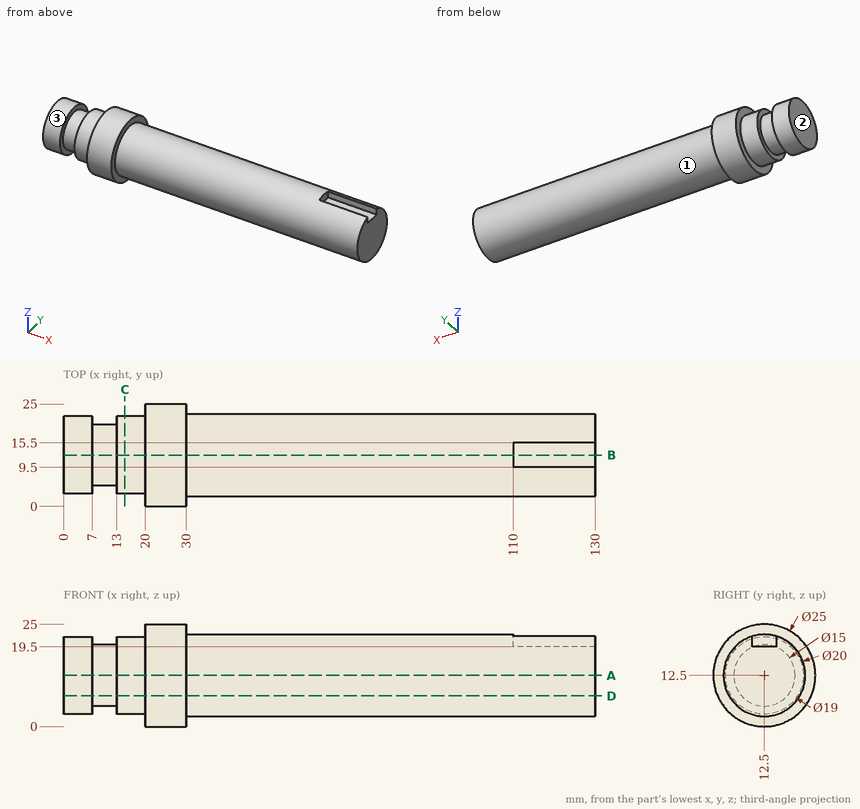
Here's the drawing with two shaded views (mm, measured from the low corner). I have some questions. A direction names the side the tool comes from. Coordinates: 2 decimals unless noted, no trailing zeros. Order: outer loops, then holes, each group sorted by start corner. A loop starts at its lowest first (then second) coordinate and runs counter-clockwise, first axis right, second up. Notation, with made-up numbers: (73.5, -23.5) - (84.5, -23.5) arc R28 ccw to (84.5, -1.5) - close; hole circle Ø4 at (86, 81.25). An arc over 180 degrees is marked (long way). Answer in a Markdown table with one row per item. Add a question column.
(1) If we section it at B-B, the plane y = 12.5: Please give me the cut outline in (x, z).
(2) If we section it at A-A, the plane z = 12.5: Please give me the cut outline in (x, y), then the cut area to 3 significant figures.
(3) If we section it at D-D, the plane z = 7.5: Please give me the cut outline in (x, y), then the cut area to 3 significant figures.
(4) I need wall thicknesses on L1, parallel to X at y = 9.5, z = 3.75; L2, parallel to Y at x = 118, z = 12.5; L3, parallel to X at y = 19, z = 20.5. Which ranges of each line are inside material? Lowest first, please.
(5) Will these pins go through, and if not, where does the flat tip stop? pin 1 (3 mm diameter, centred on x = 100, y = 14.5, fed in from +Z); pin 2 (3 mm diameter, centred on x = 109, z = 17.5, fed in from +Y); pin 3 (0.8 mm diameter, centred on x = 124, z = 21, fed in from -Y).
(6) On a 3-axis mill with a long thin cutter (end or side, diameter ignored), from which of +Z, -Z, +X, -X, +Y, -Y can I reach the whole of each face in a straight line? I mean the marked faces 1, 2 and 3. Say none if no direction works.
(7) If we section it at C-C, the plane x = 15: Please give me the cut outline in (y, z).
Results are:
| question | item | result |
|---|---|---|
| 1 | outline | (0, 3) - (7, 3) - (7, 5) - (13, 5) - (13, 3) - (20, 3) - (20, 0) - (30, 0) - (30, 2.5) - (130, 2.5) - (130, 19.5) - (110, 19.5) - (110, 22.5) - (30, 22.5) - (30, 25) - (20, 25) - (20, 22) - (13, 22) - (13, 20) - (7, 20) - (7, 22) - (0, 22) - close |
| 2 | outline | (0, 3) - (7, 3) - (7, 5) - (13, 5) - (13, 3) - (20, 3) - (20, 0) - (30, 0) - (30, 2.5) - (130, 2.5) - (130, 22.5) - (30, 22.5) - (30, 25) - (20, 25) - (20, 22) - (13, 22) - (13, 20) - (7, 20) - (7, 22) - (0, 22) - close |
| 2 | area | 2,610 mm2 |
| 3 | outline | (0, 4.42) - (7, 4.42) - (7, 6.91) - (13, 6.91) - (13, 4.42) - (20, 4.42) - (20, 1.04) - (30, 1.04) - (30, 3.84) - (130, 3.84) - (130, 21.16) - (30, 21.16) - (30, 23.96) - (20, 23.96) - (20, 20.58) - (13, 20.58) - (13, 18.09) - (7, 18.09) - (7, 20.58) - (0, 20.58) - close |
| 3 | area | 2,250 mm2 |
| 4 | L1 | x = 0 to 7, 13 to 130 |
| 4 | L2 | y = 2.5 to 22.5 |
| 4 | L3 | x = 20 to 30 |
| 5 | pin 1 | stops at z = 22.49 |
| 5 | pin 2 | stops at y = 21.87 |
| 5 | pin 3 | stops at y = 6.64 |
| 6 | face 1 | +X |
| 6 | face 2 | +Z, -Z, -X, +Y, -Y |
| 6 | face 3 | -X |
| 7 | outline | circle Ø19 at (12.5, 12.5) |
